from build123d import *

# Parameters (mm, degrees)
BOSS_EXTRUDE1_DEPTH      = 56
SHELL1_T                 = -4
CUT_EXTRUDE1_START       = -4
SKETCH2_R                = 6.25
CUT_EXTRUDE1_DEPTH       = 2
CUT_EXTRUDE2_START       = -54
SKETCH2_2_R              = 6.25
CUT_EXTRUDE2_DEPTH       = 2
BOSS_EXTRUDE2_DEPTH      = 4
BOSS_EXTRUDE2_DEPTH_BACK = 1
SKETCH3_W                = 54
SKETCH3_H                = 25
BOSS_EXTRUDE3_DEPTH      = 5
BOSS_EXTRUDE4_START      = -49
BOSS_EXTRUDE4_DEPTH      = 5


with BuildPart() as part:
    # Sketch1 → Boss-Extrude1 (new body)
    with BuildSketch(Plane(origin=(0, 0, 0), x_dir=(1, 0, 0), z_dir=(0, 1, 0))):
        with BuildLine():
            Line((0, 0), (0, 16))
            Line((0, 16), (18.828724193, 16))
            ThreePointArc((18.828724193, 16), (26.828724193, 8), (18.828724193, 0))
            Line((18.828724193, 0), (0, 0))
        make_face()
    extrude(amount=BOSS_EXTRUDE1_DEPTH)

    # Shell1
    shell1_openings = [part.faces().sort_by_distance(p)[0] for p in [
        (9.414362096, 28, 0),
        (9.414362096, 28, -16),
        (26.828724193, 28, -8),
    ]]
    offset(amount=SHELL1_T, openings=shell1_openings, kind=Kind.INTERSECTION)

    # Sketch2 → Cut-Extrude1 (cut)
    with BuildSketch(Plane.XZ.offset(CUT_EXTRUDE1_START)):
        with Locations(Location((18.828724193, -8, 0), (0, 0, 90))):
            Circle(SKETCH2_R)
    extrude(amount=CUT_EXTRUDE1_DEPTH, mode=Mode.SUBTRACT)

    # Sketch2<2> → Cut-Extrude2 (cut)
    with BuildSketch(Plane.XZ.offset(CUT_EXTRUDE2_START)):
        with Locations(Location((18.828724193, -8, 0), (0, 0, 90))):
            Circle(SKETCH2_2_R)
    extrude(amount=CUT_EXTRUDE2_DEPTH, mode=Mode.SUBTRACT)

    # Sketch3 → Boss-Extrude2 (add, two sides: drawn at the far end of the back side and taken through both)
    with BuildSketch(Plane.ZY.offset(-BOSS_EXTRUDE2_DEPTH_BACK)):
        with Locations((-8, 28)):
            Rectangle(SKETCH3_W, SKETCH3_H)
    extrude(amount=BOSS_EXTRUDE2_DEPTH + BOSS_EXTRUDE2_DEPTH_BACK)

    # Sketch4 → Boss-Extrude3 (add)
    with BuildSketch(Plane.XY.offset(19)):
        with BuildLine():
            Line((-4, 15.5), (-4, 40.5))
            Line((-4, 40.5), (-22, 40.5))
            ThreePointArc((-22, 40.5), (-26, 28), (-22, 15.5))
            Line((-22, 15.5), (-4, 15.5))
        make_face()
    extrude(amount=-BOSS_EXTRUDE3_DEPTH)

    # Sketch4<4> → Boss-Extrude4 (add)
    with BuildSketch(Plane.XY.offset(19).offset(BOSS_EXTRUDE4_START)):
        with BuildLine():
            Line((-4, 15.5), (-4, 40.5))
            Line((-4, 40.5), (-22, 40.5))
            ThreePointArc((-22, 40.5), (-26, 28), (-22, 15.5))
            Line((-22, 15.5), (-4, 15.5))
        make_face()
    extrude(amount=-BOSS_EXTRUDE4_DEPTH)


solid = part.part
Source: CAD feature listing. Evaluate the final solid. Frame: model axes, mm. A direction names the side the tool comes from. Give positions to 0.01 mm unless a question says otherwise; leave off trailing zeros. Write each loop counter-clockwise with the first axis right and the second up, starting at its lowest first coordinate (ties: lowest second). Pieces come first, ordered by that corner, then holes. Notation, with made-up numbers: M 55,58.5 L 80,58.5 A26 cw 80,84.5 Z; hole C -26.5,33 d3. An arc over 180 degrees is marked long. Return JSON: item names as keys, results as strings. Group by question number.
1) Pin query (flat end, axial travel): P1, Ø15, axis at x = 11, y = 37, coming from the +Z side; P2, Ø7, axis at x = -9, z = -3, coming from the +Y side; P3, Ø21, axis at y = 22.5, z = -22, coming from the +X side; P4, Ø5, axis at y = 34, z = 4.5, coming from the +X side. Return the tip coordinate at first contact, or that it passes through.
2) Material intervals for line 1 along Z through (x, y) = (-18.5, 34.5); line 2 along X through (y, z) = (52.6, -8); line 3 along Y through (x, z) = (23, -5), sorted ascending. Write a range as [from, to].
3) Set-up query: faces 4 (the face through (-15, 28, 14)), 5 (the face through (1, 28, 9)), 6 (the face through (19, 2, -8)), 7 (the face through (0, 8, -8)). Return all of +Z, -Z, +X, -X, +Y, -Y with unobstructed straight access to the full face (end or side cutting, diameter ignored); none if empty.
4) Cut plane C-C, the plane y = 46.5. Output: boundary loops of the cut face in (x, z), plus the area to 3 significant figures.
5) Cut plane D-D, the plane x = -12.5. Output: boundary loops of the cut face in (y, z), plus the area to 3 significant figures.
6) Cut plane A-A, the plane x = 9.5. Output: boundary loops of the cut face in (y, z), plus the area to 3 significant figures.
7) Cut plane B-B, the plane z = -8. Output: boundary loops of the cut face in (x, y).
8) Pull-direction query (X, two-part tool) for faces 1 (the face through (0, 48, -8)), 2 (the face through (25, 3, -9)), 3 (the face through (4, 28, -8)); classes: pulls with the +X half, pulls with the -X half, needs draft (parallel to the pull), parting line crosses it, or undercut.
Recorded:
{
 "1": {"P1": "stops at z = 0", "P2": "passes through", "P3": "stops at x = 4", "P4": "stops at x = 1"},
 "2": {"line 1": "z = [-35, -30], [14, 19]", "line 2": "x = [0, 12.58], [25.08, 26.83]", "line 3": "y = [0, 2], [54, 56]"},
 "3": {"face 4": "-X, +Y, -Y", "face 5": "+Z, +X, +Y, -Y", "face 6": "none", "face 7": "+Z, -Z, -X, -Y"},
 "4": {"outline": "M 0,-16 L 4,-16 L 4,0 L 0,0 Z", "area": "64.0 mm²"},
 "5": {"outline": "M 15.5,-35 L 40.5,-35 L 40.5,-30 L 15.5,-30 Z; M 15.5,14 L 40.5,14 L 40.5,19 L 15.5,19 Z", "area": "250 mm²"},
 "6": {"outline": "M 0,-16 L 4,-16 L 4,0 L 0,0 Z; M 52,-16 L 56,-16 L 56,0 L 52,0 Z", "area": "128 mm²"},
 "7": {"outline": "M -4,15.5 L 0,15.5 L 0,0 L 26.83,0 L 26.83,4 L 25.08,4 L 25.08,2 L 12.58,2 L 12.58,4 L 4,4 L 4,52 L 12.58,52 L 12.58,54 L 25.08,54 L 25.08,52 L 26.83,52 L 26.83,56 L 0,56 L 0,40.5 L -4,40.5 Z"},
 "8": {"face 1": "pulls with the -X half", "face 2": "undercut", "face 3": "pulls with the +X half"}
}
